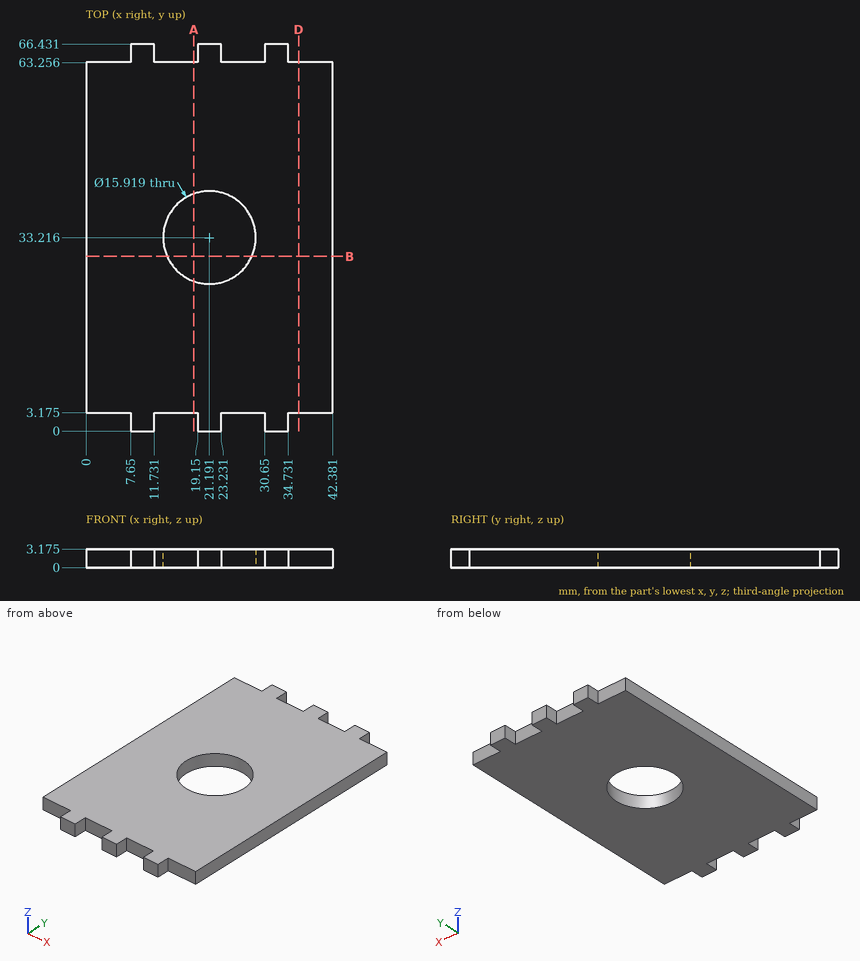
Job drawing, mm, ordinate dimensions from the low corner. One solid piece. Round coordinates to 2 decimals unless told otherwise and drop trailing zeros. Loops run counter-clockwise (first coordinate to the right, second up) from the corner with the lowest first, then second, coordinate; pieces in that order, holes last. Notation, with made-up numbers: M 73,14.25 L 110,14.25 A14 cw 110,18.25 Z; hole C 29.25,17 d11. An arc over 180 degrees is marked long. Answer as CSV lines item,"result".
1. Cut at B-B on y = 30. Write the cut outline in (x, z) (1 decimal).
Resolved:
outline,"M 0,0 L 13.9,0 L 13.9,3.2 L 0,3.2 Z; M 28.5,0 L 42.4,0 L 42.4,3.2 L 28.5,3.2 Z"
2. Wall check: probe 1 along X at (y, z) = (3, 0.45); probe 2 along Y at (x, z) = (37, 1.4) (1 decimal); probe 3 along Y at (x, z) = (21.5, 2.45). Give the ranges that are in metal, low to high. Write a range as [from, to].
Resolved:
probe 1,"x = [7.65, 11.73], [19.15, 23.23], [30.65, 34.73]"
probe 2,"y = [3.2, 63.3]"
probe 3,"y = [0, 25.26], [41.17, 66.43]"
3. Flat gauge pins, fed straight in: P1, Ø1.6, axis at x = 26.5, z = 1.5, coming from the +Y side; P2, Ø1, axis at y = 1.5, z = 2, coming from the -X side; P3, Ø1.6, axis at y = 1, z = 1.5, coming from the +X side. Where does each tip first touch, or does it go through?
Resolved:
P1,"stops at y = 63.26"
P2,"stops at x = 7.65"
P3,"stops at x = 34.73"
4. Cut at A-A on x = 18.5. Write the cut outline in (y, z) (1 decimal).
Resolved:
outline,"M 3.2,0 L 25.7,0 L 25.7,3.2 L 3.2,3.2 Z; M 40.7,0 L 63.3,0 L 63.3,3.2 L 40.7,3.2 Z"
5. Cut at D-D on x = 36.5. Write the cut outline in (y, z) (1 decimal), then the cut area to 3 significant figures.
Resolved:
outline,"M 3.2,0 L 63.3,0 L 63.3,3.2 L 3.2,3.2 Z"
area,"191 mm²"
